Can you work these out from the drawing? Everything is in mm from the part's minimum corner. A direction names the side the tool comes from. Round coordinates to 2 decimals unless told otherwise and drop trailing zeros. Write each loop counter-clockwise with the first axis right and the second up, starting at its lowest first coordinate (ties: lowest second). Pieces come first, ordered by that corner, then holes. Notation, with made-up numbers: M 5.25,64.25 L 35.25,64.25 A19 ccw 35.25,100.25 Z; hole C 89.5,63 d9. An arc over 180 degrees is marked long. Use one line per item in the form item = value. Start each with the question number.
Q1. I want a section at D-D on x = 14. List the corners of the cut face in (y, z) for me, and give its area (3 significant figures).
Q2. I want a section at C-C on y = 5. List the corners of the cut face in (x, z) for me, and give its area (3 significant figures).
Q3. I want a section at B-B on z = 2.05. List the corners of the cut face in (x, y) for me.
Q4. I need wall thicknesses on line 1 along X through (y, z) = (7.75, 0.7); line 2 along Y through (x, z) = (9, 1.75); line 3 along X through (y, z) = (1, 1.8). Which ranges of each line are inside material? Lowest first, please. Write a range as from..to.
Q5. For the marked faces 1 and 2, which set-ups out of +Z, -Z, +X, -X, +Y, -Y let a thin tool reach every point of the face, with its end or its side?
Q6. We'd pull the mould along X, two halves only. Please class the marked faces 3, 4, 5 and 6: +X half, -X half, draft (parallel to the pull), parting line (faces both ways), or undercut.
Q7. I want a section at A-A on x = 9. List the corners of the cut face in (y, z) for me.
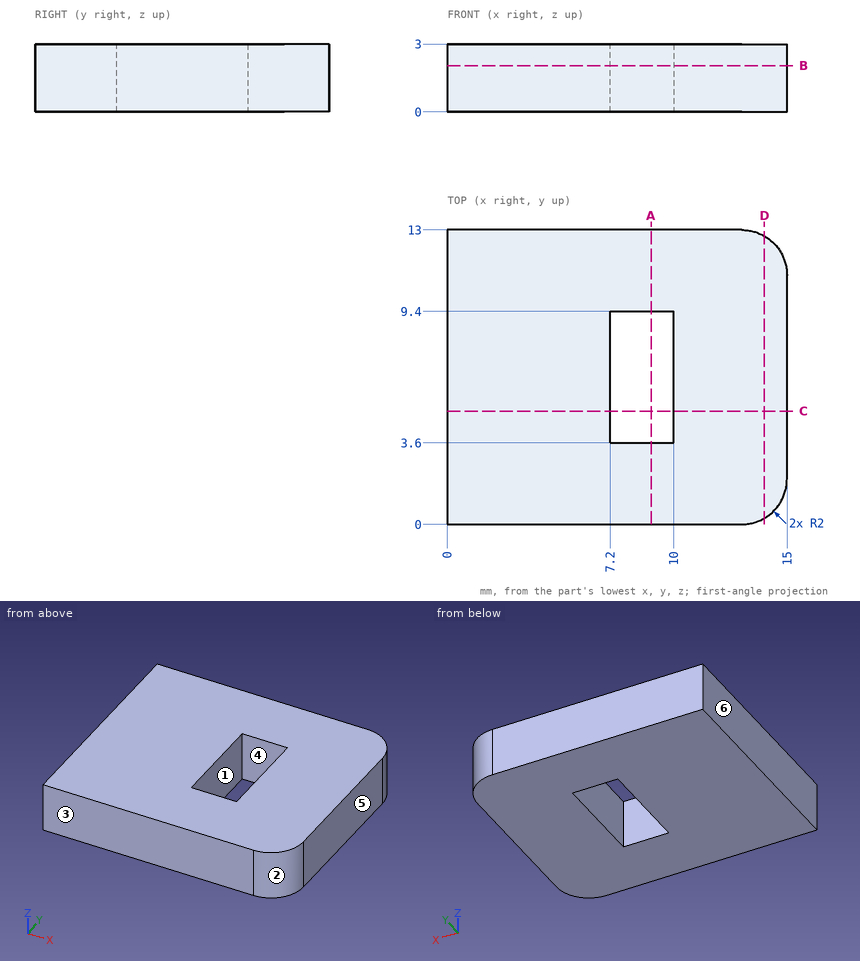
Reported:
q1.outline = M 0.27,0 L 12.73,0 L 12.73,3 L 0.27,3 Z
q1.area = 37.4 mm^2
q2.outline = M 0,0 L 7.2,0 L 7.2,3 L 0,3 Z; M 10,0 L 15,0 L 15,3 L 10,3 Z
q2.area = 36.6 mm^2
q3.outline = M 0,0 L 13,0 A2 ccw 15,2 L 15,11 A2 ccw 13,13 L 0,13 Z; hole M 7.2,3.6 L 10,3.6 L 10,9.4 L 7.2,9.4 Z
q4.line_1 = 0..7.2, 10..15
q4.line_2 = 0..3.6, 9.4..13
q4.line_3 = 0..14.73
q5.face_1 = +Z, -Z
q5.face_2 = +Z, -Z, +X, -Y
q6.face_3 = draft
q6.face_4 = undercut
q6.face_5 = +X half
q6.face_6 = -X half
q7.outline = M 0,0 L 3.6,0 L 3.6,3 L 0,3 Z; M 9.4,0 L 13,0 L 13,3 L 9.4,3 Z
